Input: part model. Units: mm. Frame: model coordinates. Give positions to 0.01 mm unless a question says otherwise; leave off trailing zeros. Loops run counter-clockwise (first coordinate to the right, second up) from the corner with the lowest first, then second, coordinate; pieces in that order, holes last. Notation, with made-up numbers: (-14, -29) - (11, -29) arc R21 ccw to (11, -22) - close; hole circle Ø11 at (1, -10). An arc over 180 degrees is marked (long way). One line per item, written item: value.
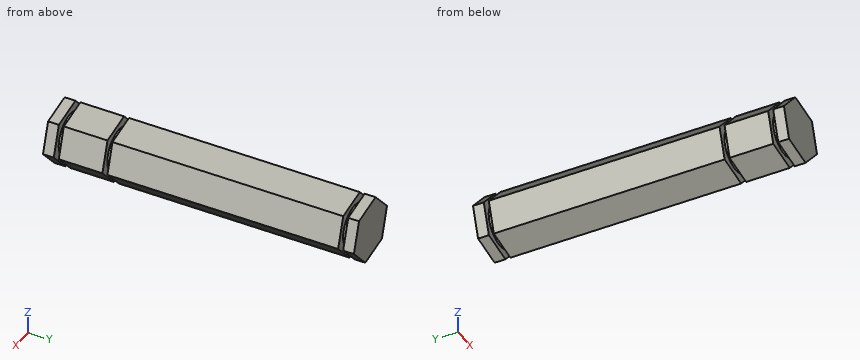
from build123d import *

# Parameters (mm, degrees)
BOSS_EXTRUDE1_DEPTH = 54.356
SKETCH2_R           = 5.0292
BOSS_EXTRUDE2_DEPTH = 1.1684
BOSS_EXTRUDE3_DEPTH = 2.54
BOSS_EXTRUDE4_START = 1.1684
SKETCH4_R           = 5.0292
BOSS_EXTRUDE4_DEPTH = 1.1684
BOSS_EXTRUDE5_DEPTH = 10.287
BOSS_EXTRUDE6_START = 1.1684
SKETCH6_R           = 5.0292
BOSS_EXTRUDE6_DEPTH = 1.1684
BOSS_EXTRUDE7_DEPTH = 2.54


with BuildPart() as part:
    # Sketch1 → Boss-Extrude1 (new body)
    with BuildSketch(Plane(origin=(0, 0, 0), x_dir=(1, 0, 0), z_dir=(0, 1, 0))):
        Polygon((4.957467016, -5.40248592), (7.157423558, 1.592049415), (2.199956542, 6.994535335), (-4.957467016, 5.40248592), (-7.157423558, -1.592049415), (-2.199956542, -6.994535335), align=None)
    extrude(amount=BOSS_EXTRUDE1_DEPTH)

    # Sketch2 → Boss-Extrude2 (add)
    with BuildSketch(Plane(origin=(0, 54.356, 0), x_dir=(1, 0, 0), z_dir=(0, 1, 0))):
        with Locations(Location((0, 0, 0), (0, 0, 270))):
            Circle(SKETCH2_R)
    extrude(amount=BOSS_EXTRUDE2_DEPTH)

    # Sketch3 → Boss-Extrude3 (add)
    with BuildSketch(Plane(origin=(0, 55.5244, 0), x_dir=(1, 0, 0), z_dir=(0, 1, 0))):
        Polygon((-2.199956542, -6.994535335), (4.957467016, -5.40248592), (7.157423558, 1.592049415), (2.199956542, 6.994535335), (-4.957467016, 5.40248592), (-7.157423558, -1.592049415), align=None)
    extrude(amount=BOSS_EXTRUDE3_DEPTH)

    # Sketch4 → Boss-Extrude4 (add)
    with BuildSketch(Plane.XZ.offset(BOSS_EXTRUDE4_START)):
        with Locations(Location((0, 0, 0), (0, 0, 90))):
            Circle(SKETCH4_R)
    extrude(amount=-BOSS_EXTRUDE4_DEPTH)

    # Sketch5 → Boss-Extrude5 (add)
    with BuildSketch(Plane.XZ.offset(1.1684)):
        Polygon((4.957467016, 5.40248592), (-2.199956542, 6.994535335), (-7.157423558, 1.592049415), (-4.957467016, -5.40248592), (2.199956542, -6.994535335), (7.157423558, -1.592049415), align=None)
    extrude(amount=BOSS_EXTRUDE5_DEPTH)

    # Sketch6 → Boss-Extrude6 (add)
    with BuildSketch(Plane.XZ.offset(11.4554).offset(BOSS_EXTRUDE6_START)):
        with Locations(Location((0, 0, 0), (0, 0, 90))):
            Circle(SKETCH6_R)
    extrude(amount=-BOSS_EXTRUDE6_DEPTH)

    # Sketch7 → Boss-Extrude7 (add)
    with BuildSketch(Plane.XZ.offset(12.6238)):
        Polygon((7.157423558, -1.592049415), (4.957467016, 5.40248592), (-2.199956542, 6.994535335), (-7.157423558, 1.592049415), (-4.957467016, -5.40248592), (2.199956542, -6.994535335), align=None)
    extrude(amount=BOSS_EXTRUDE7_DEPTH)


solid = part.part
Item 1: Section A-A, the plane x = 6. Output: boundary loops of the cut face in (y, z).
Verdict:
outline: (-15.16, -2.85) - (-12.62, -2.85) - (-12.62, 2.09) - (-15.16, 2.09) - close; (-11.46, -2.85) - (-1.17, -2.85) - (-1.17, 2.09) - (-11.46, 2.09) - close; (0, -2.85) - (54.36, -2.85) - (54.36, 2.09) - (0, 2.09) - close; (55.52, -2.85) - (58.06, -2.85) - (58.06, 2.09) - (55.52, 2.09) - close
Item 2: Material intervals for L1, parallel to Y at x = -2.75, z = -4.25; L2, parallel to Z at x = 0.75, y = 4; L3, parallel to Z at x = -4.75, y = -4, sorted ascending.
Verdict:
L1: y = -15.16 to -12.62, -11.46 to -1.17, 0 to 54.36, 55.52 to 58.06
L2: z = -6.67 to 6.34
L3: z = -5.45 to 4.22
Item 3: Pin query (flat end, axial travel): P1, Ø1, axis at y = 13.5, z = 0.5, coming from the -X side. Return the tip coordinate at first contact, or that it passes through.
Verdict:
P1: stops at x = -6.97
Item 4: Section C-C, the plane y = 50. Output: boundary loops of the cut face in (x, z).
Verdict:
outline: (-7.16, 1.59) - (-4.96, -5.4) - (2.2, -6.99) - (7.16, -1.59) - (4.96, 5.4) - (-2.2, 6.99) - close
Item 5: Section B-B, the plane z = -2.5. Output: boundary loops of the cut face in (x, y), and give its area (3 significant figures).
Verdict:
outline: (-5.87, -15.16) - (6.32, -15.16) - (6.32, -12.62) - (4.36, -12.62) - (4.36, -11.46) - (6.32, -11.46) - (6.32, -1.17) - (4.36, -1.17) - (4.36, 0) - (6.32, 0) - (6.32, 54.36) - (4.36, 54.36) - (4.36, 55.52) - (6.32, 55.52) - (6.32, 58.06) - (-5.87, 58.06) - (-5.87, 55.52) - (-4.36, 55.52) - (-4.36, 54.36) - (-5.87, 54.36) - (-5.87, 0) - (-4.36, 0) - (-4.36, -1.17) - (-5.87, -1.17) - (-5.87, -11.46) - (-4.36, -11.46) - (-4.36, -12.62) - (-5.87, -12.62) - close
area: 881 mm^2
Item 6: Section D-D, the plane x = 1.25. Output: boundary loops of the cut face in (y, z).
Verdict:
outline: (-15.16, -6.78) - (-12.62, -6.78) - (-12.62, -4.87) - (-11.46, -4.87) - (-11.46, -6.78) - (-1.17, -6.78) - (-1.17, -4.87) - (0, -4.87) - (0, -6.78) - (54.36, -6.78) - (54.36, -4.87) - (55.52, -4.87) - (55.52, -6.78) - (58.06, -6.78) - (58.06, 6.23) - (55.52, 6.23) - (55.52, 4.87) - (54.36, 4.87) - (54.36, 6.23) - (0, 6.23) - (0, 4.87) - (-1.17, 4.87) - (-1.17, 6.23) - (-11.46, 6.23) - (-11.46, 4.87) - (-12.62, 4.87) - (-12.62, 6.23) - (-15.16, 6.23) - close
